Check sheet for the modelled part. Datum: model origin and axes. Units: mm. Coordinates: 2 decimals unless noted, no trailing zeros. Write each loop counter-clockwise with the first axis right and the second up, starting at its lowest first coordinate (ties: lowest second). Pieces come first, ordered by that corner, then holes. Notation, with made-up numbers: (-3.75, 49) - (6.25, 49) arc R17 ccw to (6.25, 63) - close; hole circle Ø3 at (-17, 2.25). An arc over 180 degrees is marked (long way). Write each question's results on one line, items separated by ' | '.
from build123d import *

# Parameters (mm, degrees)
F1_DEPTH = 304.8
F2_DEPTH = 38.1
F4_DEPTH = 38.1


with BuildPart() as f1:
    # F0 (on Front) → F1 (new body)
    with BuildSketch(Plane.XZ):
        with BuildLine():
            Line((-43.809108, 25.717738), (-55.269517, 25.717738))
            ThreePointArc((-55.269517, 25.717738), (-60.96, 0), (-55.269517, -25.717738))
            Line((-55.269517, -25.717738), (-43.809108, -25.717738))
            ThreePointArc((-43.809108, -25.717738), (-50.8, 0), (-43.809108, 25.717738))
        make_face()
        with BuildLine():
            ThreePointArc((55.269517, -25.717738), (59.52038, -13.169887), (60.96, 0))
            ThreePointArc((60.96, 0), (59.52038, 13.169887), (55.269517, 25.717738))
            Line((55.269517, 25.717738), (43.809108, 25.717738))
            ThreePointArc((43.809108, 25.717738), (49.021132, 13.325489), (50.8, 0))
            ThreePointArc((50.8, 0), (49.021132, -13.325489), (43.809108, -25.717738))
            Line((43.809108, -25.717738), (55.269517, -25.717738))
        make_face()
    extrude(amount=F1_DEPTH)

    # F0 (on Front) → F2 (join)
    with BuildSketch(Plane.XZ):
        with BuildLine():
            Line((43.809108, 25.717738), (55.269517, 25.717738))
            ThreePointArc((55.269517, 25.717738), (0, 60.96), (-55.269517, 25.717738))
            Line((-55.269517, 25.717738), (-43.809108, 25.717738))
            ThreePointArc((-43.809108, 25.717738), (0, 50.8), (43.809108, 25.717738))
        make_face()
        with BuildLine():
            ThreePointArc((-55.269517, -25.717738), (0, -60.96), (55.269517, -25.717738))
            Line((55.269517, -25.717738), (43.809108, -25.717738))
            ThreePointArc((43.809108, -25.717738), (0, -50.8), (-43.809108, -25.717738))
            Line((-43.809108, -25.717738), (-55.269517, -25.717738))
        make_face()
    extrude(amount=F2_DEPTH)

    # F3 (on face) → F4 (join)
    with BuildSketch(Plane.XZ.offset(304.8)):
        with BuildLine():
            Line((-43.809108, 25.717738), (-55.269517, 25.717738))
            ThreePointArc((-55.269517, 25.717738), (-60.96, 0), (-55.269517, -25.717738))
            Line((-55.269517, -25.717738), (-43.809108, -25.717738))
            ThreePointArc((-43.809108, -25.717738), (-50.8, 0), (-43.809108, 25.717738))
        make_face()
        with BuildLine():
            ThreePointArc((-55.269517, -25.717738), (13.169887, -59.52038), (60.96, 0))
            ThreePointArc((60.96, 0), (13.169887, 59.52038), (-55.269517, 25.717738))
            Line((-55.269517, 25.717738), (-43.809108, 25.717738))
            ThreePointArc((-43.809108, 25.717738), (13.325489, 49.021132), (50.8, 0))
            ThreePointArc((50.8, 0), (13.325489, -49.021132), (-43.809108, -25.717738))
            Line((-43.809108, -25.717738), (-55.269517, -25.717738))
        make_face()
    extrude(amount=F4_DEPTH)


solid = f1.part
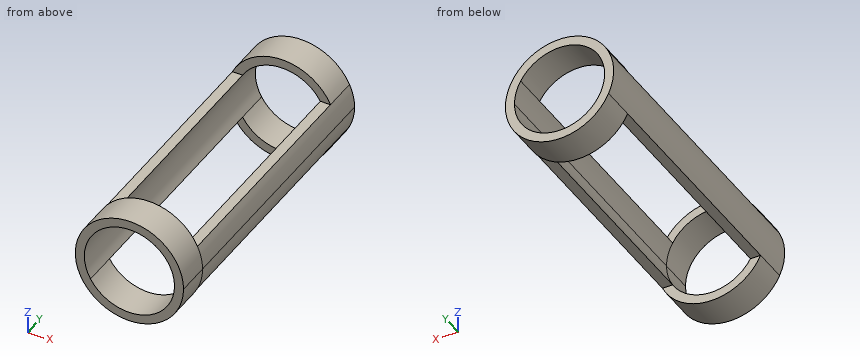
1. Go/stop test with flat-tipped pins: pin 1 (12 mm diameter, centred on y = -54, z = -11, fed in from -X); pin 2 (1 mm diameter, centred on y = -206, z = 21, fed in from -X); pin 3 (9 mm diameter, centred on x = 52.5, y = -119.5, fed in from +Z). Record where each tip stops, or that it passes through.
Values follow:
pin 1: stops at x = -60.75 | pin 2: stops at x = -57.41 | pin 3: stops at z = 25.72
2. Material ranges on L1, parallel to X at y = -222, z = -2.5; L2, parallel to X at y = -103, z = 18; L3, parallel to Y at x = 48, z = 36.5, recorded low to high. Write a range as [from, to].
Values follow:
L1: x = [-60.91, -50.74], [50.74, 60.91] | L2: x = [-58.24, -47.5], [47.5, 58.24] | L3: y = [-342.9, -304.8], [-38.1, 0]
3. Sectioned sample at A-A (y = -271). Record the cut outline in (x, z), then the cut area to 3 significant figures.
Values follow:
outline: (-55.27, -25.72) - (-43.81, -25.72) arc R50.8 cw to (-43.81, 25.72) - (-55.27, 25.72) arc R60.96 ccw to start; (43.81, -25.72) - (55.27, -25.72) arc R60.96 ccw to (60.96, 0) arc R60.96 ccw to (55.27, 25.72) - (43.81, 25.72) arc R50.8 cw to (50.8, 0) arc R50.8 cw to start | area: 1,090 mm^2
4. Sectioned sample at C-C (y = -21). Record the cut outline in (x, z).
Values follow:
outline: (-55.27, -25.72) arc R60.96 ccw to (55.27, -25.72) arc R60.96 ccw to (60.96, 0) arc R60.96 ccw to (55.27, 25.72) arc R60.96 ccw to (-55.27, 25.72) arc R60.96 ccw to start; hole (43.81, -25.72) arc R50.8 ccw to (50.8, 0) arc R50.8 ccw to (43.81, 25.72) arc R50.8 ccw (long way) to start
5. Sectioned sample at B-B (x = 20). Record the cut outline in (y, z), then the cut area to 3 significant figures.
Values follow:
outline: (-342.9, -57.59) - (-304.8, -57.59) - (-304.8, -46.7) - (-342.9, -46.7) - close; (-342.9, 46.7) - (-304.8, 46.7) - (-304.8, 57.59) - (-342.9, 57.59) - close; (-38.1, -57.59) - (0, -57.59) - (0, -46.7) - (-38.1, -46.7) - close; (-38.1, 46.7) - (0, 46.7) - (0, 57.59) - (-38.1, 57.59) - close | area: 1,660 mm^2
6. Sectioned sample at D-D (z = -19). Record the cut outline in (x, y), then the cut area to 3 significant figures.
Values follow:
outline: (-57.92, -342.9) - (-47.11, -342.9) - (-47.11, 0) - (-57.92, 0) - close; (47.11, -342.9) - (57.92, -342.9) - (57.92, 0) - (47.11, 0) - close | area: 7,410 mm^2
